Could you check a few things on this model? Use its own coordinates, in mm. Round coordinates to 2 decimals unless told otherwise and drop trailing zeros. Loops run counter-clockwise (first coordinate to the right, second up) from the corner with the lowest first, then second, coordinate; pieces in that order, holes last. Notation, with made-up numbers: M 84,80 L 137,80 A25 cw 137,104 Z; hole C 45,61.25 d9. An arc over 180 degrees is marked long. Return JSON: item names as keys, results as strings. Group by question number.
Solid Edge part; units mm, degrees
sketch "Sketch1" plane through (0, 0, 0) normal (0, 0, 1) x (1, 0, 0)
  line L0 (-25, -12.5) -> (25, -12.5)
  line L1 (25, -12.5) -> (25, 12.5)
  line L2 (25, 12.5) -> (-25, 12.5)
  line L3 (-25, 12.5) -> (-25, -12.5)
  dimension "D1" = 25
extrude "Protrusion1" add sketch "Sketch1" along normal blind 6
hole "Hole_1" at (-13, 0, 6) direction (0, 0, -1) diameter 16 end up to next
hole "Hole1" at (13, 0, 6) direction (0, 0, -1) diameter 16 end up to next
1. If we section it at B-B, the plane y = 0: Please give me the cut outline in (x, z), then the cut area to 3 significant figures.
2. If we section it at D-D, the plane y = 5.5: Please give me the cut outline in (x, z), then the cut area to 3 significant figures.
3. We'd pull the mould along Y, two halves only. Please class faces 1 (the face through (0, -12.5, 3)), 2 (the face through (0, 0, 6)), 3 (the face through (5.19, 1.73, 3.04)): +Y half, -Y half, draft (parallel to the pull), parting line (faces both ways), or undercut.
4. I'm going to push a flat-ended pin straight in: pin 1 Ø13 at (x, y) = (-13, 0) entering from -Z. Where does the tip first touch, or does it pass through?
5. If we section it at A-A, the plane x = -13: Please give me the cut outline in (y, z), then the cut area to 3 significant figures.
6. I need wall thicknesses on probe 1 along X at (y, z) = (0, 2.55); probe 2 along X at (y, z) = (-6.25, 3.45); probe 3 along Y at (x, z) = (-13, 2.05). Which ranges of each line are inside material? Lowest first, please.
7. If we section it at C-C, the plane z = 3.3: Please give me the cut outline in (x, y), then the cut area to 3 significant figures.
Geometry results:
{
 "1": {"outline": "M -25,0 L -21,0 L -21,6 L -25,6 Z; M -5,0 L 5,0 L 5,6 L -5,6 Z; M 21,0 L 25,0 L 25,6 L 21,6 Z", "area": "108 mm^2"},
 "2": {"outline": "M -25,0 L -18.81,0 L -18.81,6 L -25,6 Z; M -7.19,0 L 7.19,0 L 7.19,6 L -7.19,6 Z; M 18.81,0 L 25,0 L 25,6 L 18.81,6 Z", "area": "161 mm^2"},
 "3": {"face 1": "-Y half", "face 2": "draft", "face 3": "undercut"},
 "4": {"pin 1": "through"},
 "5": {"outline": "M -12.5,0 L -8,0 L -8,6 L -12.5,6 Z; M 8,0 L 12.5,0 L 12.5,6 L 8,6 Z", "area": "54.0 mm^2"},
 "6": {"probe 1": "-25 to -21, -5 to 5, 21 to 25", "probe 2": "-25 to -17.99, -8.01 to 8.01, 17.99 to 25", "probe 3": "-12.5 to -8, 8 to 12.5"},
 "7": {"outline": "M -25,-12.5 L 25,-12.5 L 25,12.5 L -25,12.5 Z; hole C -13,0 d16; hole C 13,0 d16", "area": "848 mm^2"}
}
